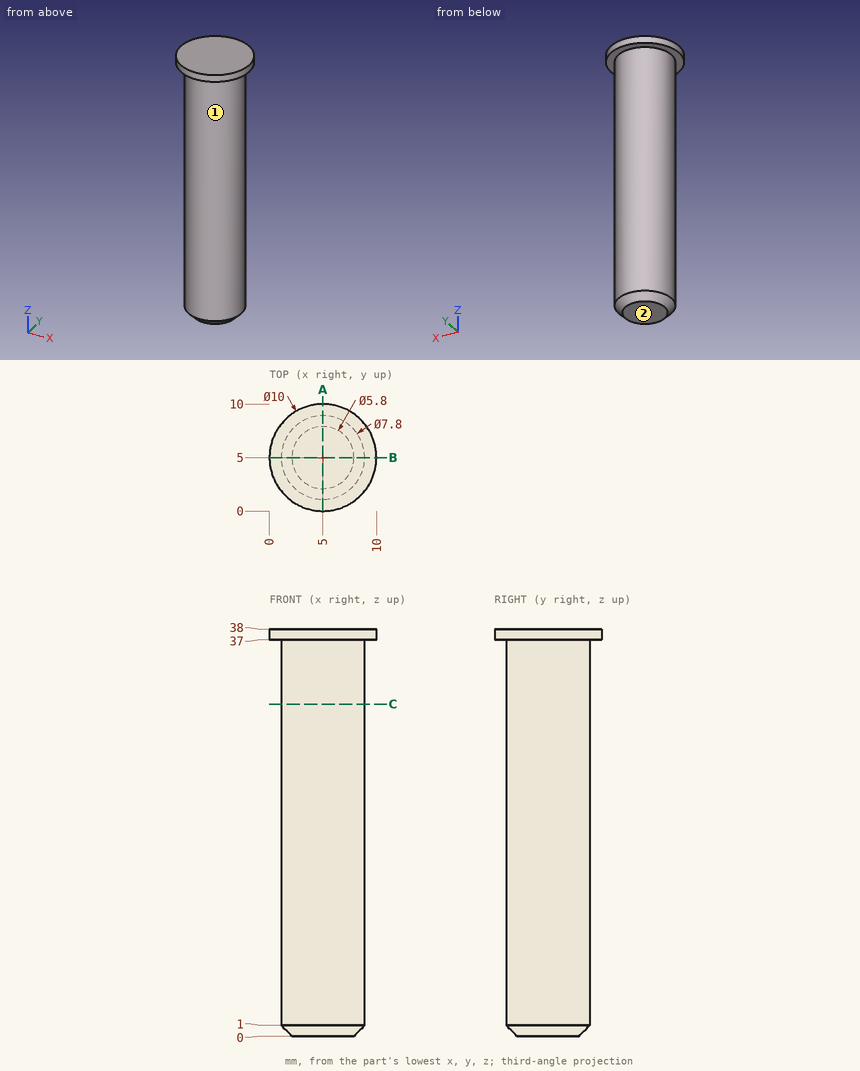
Can you work these out from the drawing? Everything is in mm from the part's minimum corner. A direction names the side the tool comes from. Coordinates: 2 decimals unless noted, no trailing zeros. Loops run counter-clockwise (first coordinate to the right, second up) from the corner with the lowest first, then second, coordinate; pieces in that order, holes last. Notation, with made-up numbers: (76, 31.25) - (91, 31.25) arc R16 cw to (91, 47.25) - close; hole circle Ø4 at (-10, 6.5). An arc over 180 degrees is marked (long way). Use a Markdown table: item, result.
Item 1: For the marked faces 1 and 2, which set-ups out of +Z, -Z, +X, -X, +Y, -Y let a thin tool reach every point of the face, with its end or its side?
Numbers:
| item | result |
|---|---|
| face 1 | -Z |
| face 2 | -Z, +X, -X, +Y, -Y |
Item 2: I want a section at A-A on x = 5. Please give me the cut outline in (y, z).
Numbers:
| item | result |
|---|---|
| outline | (0, 37) - (1.1, 37) - (1.1, 1) - (2.1, 0) - (7.9, 0) - (8.9, 1) - (8.9, 37) - (10, 37) - (10, 38) - (0, 38) - close |
Item 3: Will these pins go through, and if not, where does the flat tip stop? pin 1 (1.5 mm diameter, centred on x = 1.5, z = 26, fed in from -Y); pin 2 (5 mm diameter, centred on y = 3, z = 9, fed in from -X); pin 3 (6 mm diameter, centred on x = 1, z = 5, fed in from -Y).
Numbers:
| item | result |
|---|---|
| pin 1 | stops at y = 2.23 |
| pin 2 | stops at x = 1.1 |
| pin 3 | stops at y = 1.23 |
Item 4: I want a section at C-C on z = 31. Please give me the cut outline in (x, y).
Numbers:
| item | result |
|---|---|
| outline | circle Ø7.8 at (5, 5) |
Item 5: If I drill on probe 1 along Z at (x, y) = (6.5, 9); probe 2 along X at (y, z) = (5.25, 29); probe 3 along X at (y, z) = (7.25, 9), over which ranges is the centre line in solid material (lowest first)? Write a range as from..to.
Numbers:
| item | result |
|---|---|
| probe 1 | z = 37..38 |
| probe 2 | x = 1.11..8.89 |
| probe 3 | x = 1.81..8.19 |
